```python
from build123d import *

# Parameters (mm, degrees)
SKETCH1_R           = 1.6
SKETCH1_R_2         = 1.821636576
BOSS_EXTRUDE1_DEPTH = 2
CUT_EXTRUDE1_DEPTH  = 2
CUT_EXTRUDE2_REACH  = 91.979
SKETCH3_R           = 1.1


with BuildPart() as part:
    # Sketch1 → Boss-Extrude1 (new body)
    with BuildSketch(Plane.XY):
        with BuildLine():
            Line((-1.061078705, 5.279593922), (28.442500971, -0.155365716))
            ThreePointArc((28.442500971, -0.155365716), (31.654220711, -2.236114921), (32.453937644, -5.978455602))
            Line((32.453937644, -5.978455602), (21.584018369, -64.985614955))
            ThreePointArc((21.584018369, -64.985614955), (19.503269163, -68.197334694), (15.760928483, -68.997051628))
            Line((15.760928483, -68.997051628), (-13.742651194, -63.56209199))
            ThreePointArc((-13.742651194, -63.56209199), (-16.954370933, -61.481342785), (-17.754087867, -57.739002104))
            Line((-17.754087867, -57.739002104), (-15.96422722, -48.022776093))
            Line((-15.96422722, -48.022776093), (-39.673587654, -43.655190247))
            Line((-39.673587654, -43.655190247), (-52.939586595, -37.150402745))
            Line((-52.939586595, -37.150402745), (-54.821863672, -36.227455859))
            ThreePointArc((-54.821863672, -36.227455859), (-57.086606666, -33.986331814), (-57.537836973, -30.832272681))
            Line((-57.537836973, -30.832272681), (-53.644253203, -9.696023904))
            ThreePointArc((-53.644253203, -9.696023904), (-52.098740676, -6.909791889), (-49.184068361, -5.622786411))
            Line((-49.184068361, -5.622786411), (-47.096468931, -5.431144635))
            Line((-47.096468931, -5.431144635), (-32.383389672, -4.080482917))
            Line((-32.383389672, -4.080482917), (-8.674029238, -8.448068762))
            Line((-8.674029238, -8.448068762), (-6.884168591, 1.268157249))
            ThreePointArc((-6.884168591, 1.268157249), (-4.803419386, 4.479876988), (-1.061078705, 5.279593922))
        make_face()
        with Locations((-44.384822009, -9.109751657)):
            Circle(SKETCH1_R, mode=Mode.SUBTRACT)
        with Locations((-49.095120362, -34.67952071)):
            Circle(SKETCH1_R, mode=Mode.SUBTRACT)
        with Locations((-10.869919276, -59.007159353)):
            Circle(SKETCH1_R, mode=Mode.SUBTRACT)
        with Locations((14.699849777, -63.717457706)):
            Circle(SKETCH1_R, mode=Mode.SUBTRACT)
        Circle(SKETCH1_R_2, mode=Mode.SUBTRACT)
        with Locations((25.569769053, -4.710298353)):
            Circle(SKETCH1_R, mode=Mode.SUBTRACT)
        Polygon((-42.496595483, -38.291112185), (-41.746841807, -34.362402924), (-35.380415499, -35.577369777), (-36.130169175, -39.506079038), align=None, mode=Mode.SUBTRACT)
        Polygon((-37.458250782, -10.313833259), (-36.76371904, -6.674486931), (-30.329701085, -7.902352953), (-31.062719564, -11.743369783), (-37.458250782, -10.522848558), align=None, mode=Mode.SUBTRACT)
    extrude(amount=BOSS_EXTRUDE1_DEPTH)

    # Sketch2 → Cut-Extrude1 (cut)
    with BuildSketch(Plane.XY.offset(2)):
        Polygon((-42.631536652, -35.870200518), (-45.58189462, -35.326704554), (-45.944225262, -37.293609866), (-42.993867295, -37.83710583), align=None)
        Polygon((-40.509265624, -7.790030189), (-37.558907657, -8.333526153), (-37.921238299, -10.300431465), (-40.871596267, -9.756935501), align=None)
        Polygon((-22.908632922, -39.503426957), (-19.958274954, -40.04692292), (-20.320605596, -42.013828232), (-23.270963564, -41.470332268), align=None)
        Polygon((-17.836003926, -11.966752592), (-14.885645959, -12.510248555), (-15.247976601, -14.477153867), (-18.198334569, -13.933657903), align=None)
    extrude(amount=-CUT_EXTRUDE1_DEPTH, mode=Mode.SUBTRACT)

    # Sketch3 → Cut-Extrude2 (cut, up to next)
    with BuildSketch(Plane.XY.offset(2), mode=Mode.PRIVATE) as cut_extrude2_sk1:
        with Locations((-6.322810567, -51.696321435)):
            Circle(SKETCH3_R)
    cut_extrude2_tool1 = extrude(cut_extrude2_sk1.sketch, amount=-CUT_EXTRUDE2_REACH, mode=Mode.PRIVATE) & part.part
    # Sketch3 → Cut-Extrude2 (cut, up to next)
    with BuildSketch(Plane.XY.offset(2), mode=Mode.PRIVATE) as cut_extrude2_sk2:
        with Locations((11.126928282, -54.98634737)):
            Circle(SKETCH3_R)
    cut_extrude2_tool2 = extrude(cut_extrude2_sk2.sketch, amount=-CUT_EXTRUDE2_REACH, mode=Mode.PRIVATE) & part.part
    # Sketch3 → Cut-Extrude2 (cut, up to next)
    with BuildSketch(Plane.XY.offset(2), mode=Mode.PRIVATE) as cut_extrude2_sk3:
        with Locations(Location((19.120179881, -11.595126253, 0), (0, 0, 180))):
            Circle(SKETCH3_R)
    cut_extrude2_tool3 = extrude(cut_extrude2_sk3.sketch, amount=-CUT_EXTRUDE2_REACH, mode=Mode.PRIVATE) & part.part
    # Sketch3 → Cut-Extrude2 (cut, up to next)
    with BuildSketch(Plane.XY.offset(2), mode=Mode.PRIVATE) as cut_extrude2_sk4:
        with Locations(Location((1.64352088, -8.451235874, 0), (0, 0, 180))):
            Circle(SKETCH3_R)
    cut_extrude2_tool4 = extrude(cut_extrude2_sk4.sketch, amount=-CUT_EXTRUDE2_REACH, mode=Mode.PRIVATE) & part.part
    # Sketch3 → Cut-Extrude2 (cut, up to next)
    with BuildSketch(Plane.XY.offset(2), mode=Mode.PRIVATE) as cut_extrude2_sk5:
        Polygon((22.704393125, -53.387885203), (24.600919852, -43.088599847), (25.584372508, -43.269765168), (23.680211994, -53.606465934), align=None)
    cut_extrude2_tool5 = extrude(cut_extrude2_sk5.sketch, amount=-CUT_EXTRUDE2_REACH, mode=Mode.PRIVATE) & part.part
    # Sketch3 → Cut-Extrude2 (cut, up to next)
    with BuildSketch(Plane.XY.offset(2), mode=Mode.PRIVATE) as cut_extrude2_sk6:
        Polygon((28.479203416, -27.555228163), (27.49575076, -27.374062842), (29.36883744, -17.206045825), (30.352290096, -17.387211146), align=None)
    cut_extrude2_tool6 = extrude(cut_extrude2_sk6.sketch, amount=-CUT_EXTRUDE2_REACH, mode=Mode.PRIVATE) & part.part
    add(cut_extrude2_tool1.solids().sort_by_distance((-6.322811, -51.696321, 2))[0], mode=Mode.SUBTRACT)
    add(cut_extrude2_tool2.solids().sort_by_distance((11.126928, -54.986347, 2))[0], mode=Mode.SUBTRACT)
    add(cut_extrude2_tool3.solids().sort_by_distance((19.12018, -11.595126, 2))[0], mode=Mode.SUBTRACT)
    add(cut_extrude2_tool4.solids().sort_by_distance((1.643521, -8.451236, 2))[0], mode=Mode.SUBTRACT)
    add(cut_extrude2_tool5.solids().sort_by_distance((24.142887, -48.337611, 2))[0], mode=Mode.SUBTRACT)
    add(cut_extrude2_tool6.solids().sort_by_distance((28.92402, -22.380637, 2))[0], mode=Mode.SUBTRACT)


solid = part.part
```
For this review, take the finished solid that the model builds, in its own axes (mm). A direction names the side the tool comes from. Coordinates: 2 decimals unless noted, no trailing zeros. Loops run counter-clockwise (first coordinate to the right, second up) from the corner with the lowest first, then second, coordinate; pieces in that order, holes last.
1. Insertion check: P1, Ø3, axis at x = 19.12, y = -11.6, coming from the +Z side; P2, Ø2, axis at x = -6.32, y = -51.7, coming from the -Z side. Each pin has a flat end and moves straight along its axis. Give the tip position at first contact, or say it passes through.
2. Add section A-A, the plane z = 0.8. Count the separate pieces of the cut face and the enclosed holes in it, then the cut area to 3 significant figures.
3. For faces 5 (the cylindrical face through (-52.13, -6.94, 0.99)), 6 (the flat face through (-18.02, -12.96, 1.01)), 7 (the flat face through (-7.8, -3.7, 1)), list the 3-axis set-ups (+Z, -Z, +X, -X, +Y, -Y) from which the entire face can be reached by the end or side of a thin tool; tool diameter is ignored.
4. Add section B-B, the plane y = -26. Give the boundary of the cut face in (x, z), then the cut area to 3 significant figures.
5. For line 1 (Y direction, x = -20.5, z = 0.6); line 2 (Y direction, x = -48.5, z = 1); line 3 (X direction, y = -58, z = 1.2), list the stretches that pass through material, from the lowest coordinate up.
6. Mouldability with a two-part tool opening along Y and no side actions: class faces 1 (the flat face through (22.647, -59.216, 0.986)), 2 (the flat face through (-16.87, -52.95, 0.99)), 3 (the cylindrical face through (-4.849, 4.448, 0.986)), 4 (the flat face through (-39.38, -10.03, 1.01)) as +Y half, -Y half, draft (parallel to the pull), parting line (faces both ways), or undercut.
Result:
1. P1: stops at z = 2
1. P2: passes through
2. separate pieces: 1
2. enclosed holes: 16
2. area: 4,270 mm2
3. face 5: +Z, -Z, -X, +Y
3. face 6: +Z, -Z
3. face 7: +Z, -Z, +Y
4. outline: (-56.65, 0) - (27.75, 0) - (27.75, 2) - (-56.65, 2) - close
4. area: 169 mm2
5. line 1: y = -47.19 to -41.98, -39.95 to -6.27
5. line 2: y = -39.33 to -36.16, -33.19 to -5.56
5. line 3: x = -17.8 to -12.11, -9.63 to 22.87
6. face 1: -Y half
6. face 2: undercut
6. face 3: +Y half
6. face 4: undercut
